Geometry check sheet. Reference: drawing and pictorial views, mm from the part's lowest x, y, z. A direction names the side the tool comes from. Coordinates: 2 decimals unless noted, no trailing zeros. Loops run counter-clockwise (first coordinate to the right, second up) from the corner with the lowest first, then second, coordinate; pieces in that order, holes last. Notation, with made-up numbers: (-10, 62.5) - (20, 62.5) arc R22 ccw to (20, 74.5) - close; hole circle Ø6 at (-18, 52.25). An arc over 180 degrees is marked (long way). Use a Markdown table: item, result. Add a question column.
1) Draft check along X on the marked faces 4, 5 and 6. Enter one of: pulls with the +X half, pulls with the -X half, needs draft (parallel to the pull), parting line crosses it, or undercut.
2) Sectioned sample at D-D, the plane y = 26. Enter the section's corners in (x, z), then the cut area to 3 significant figures.
3) Sectioned sample at B-B, the plane x = 28.5. Enter the section's corners in (y, z).
4) Tool access check on the marked faces 1, 2 and 3. Record the directions out of +Z, -Z, +X, -X, +Y, -Y that give a thin tool (end or side, any length) a straight path to the whole face; none if there is none.
5) Go/stop test with flat-tipped pins: P1, Ø1.5, axis at x = 29, y = 16.5, coming from the +Z side; P2, Ø1.5, axis at x = 23, z = 2.5, coming from the +Y side; P3, Ø5, axis at y = 4.5, z = 2, coming from the +X side; P4, Ø2.5, axis at x = 6.5, y = 17.5, coming from the +Z side. Record where each tip stops, or that it passes through.
6) Thickness scan on line 1 (X direction, y = 16.5, z = 4.75); line 2 (Z direction, x = 22.5, y = 32.5); line 3 (Y direction, x = 27.5, z = 6.75). Record the ranges inside material, lowest first.
7) Sectioned sample at C-C, the plane z = 9.5. Enter the section's corners in (x, y) (3 decimals).
8) Sectioned sample at A-A, the plane y = 17.5. Enter the section's corners in (x, z), then the cut area to 3 significant figures.
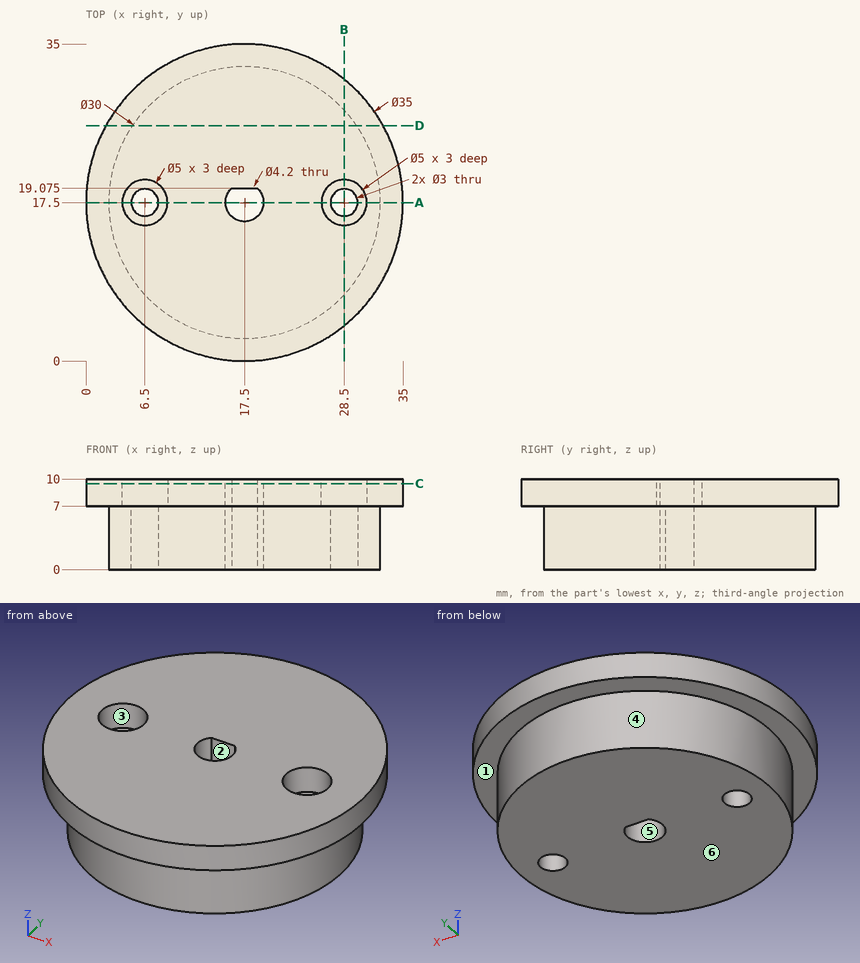
Solved:
| question | item | result |
|---|---|---|
| 1 | face 4 | parting line crosses it |
| 1 | face 5 | undercut |
| 1 | face 6 | needs draft |
| 2 | outline | (2.2, 7) - (5.14, 7) - (5.14, 0) - (29.86, 0) - (29.86, 7) - (32.8, 7) - (32.8, 10) - (2.2, 10) - close |
| 2 | area | 265 mm2 |
| 3 | outline | (3.89, 7) - (7.3, 7) - (7.3, 0) - (16, 0) - (16, 7) - (15, 7) - (15, 10) - (3.89, 10) - close; (19, 0) - (27.7, 0) - (27.7, 7) - (31.11, 7) - (31.11, 10) - (20, 10) - (20, 7) - (19, 7) - close |
| 4 | face 1 | -Z |
| 4 | face 2 | +Z, -Z |
| 4 | face 3 | +Z |
| 5 | P1 | stops at z = 7 |
| 5 | P2 | stops at y = 31.73 |
| 5 | P3 | stops at x = 28.21 |
| 5 | P4 | passes through |
| 6 | line 1 | x = 2.53 to 5.38, 7.62 to 15.65, 19.35 to 27.38, 29.62 to 32.47 |
| 6 | line 2 | z = 7 to 10 |
| 6 | line 3 | y = 6.32 to 16.38, 18.62 to 28.68 |
| 7 | outline | circle Ø35 at (17.5, 17.5); hole circle Ø5 at (6.5, 17.5); hole (16.111, 19.075) arc R2.1 ccw (long way) to (18.889, 19.075) - close; hole circle Ø5 at (28.5, 17.5) |
| 8 | outline | (0, 7) - (2.5, 7) - (2.5, 0) - (5, 0) - (5, 7) - (4, 7) - (4, 10) - (0, 10) - close; (8, 0) - (15.4, 0) - (15.4, 10) - (9, 10) - (9, 7) - (8, 7) - close; (19.6, 0) - (27, 0) - (27, 7) - (26, 7) - (26, 10) - (19.6, 10) - close; (30, 0) - (32.5, 0) - (32.5, 7) - (35, 7) - (35, 10) - (31, 10) - (31, 7) - (30, 7) - close |
| 8 | area | 201 mm2 |
